Verification items for the finished model (mm, model axes). Face numbers are marked on the shaded views. Coordinates: 2 decimals unless noted, no trailing zeros. Loops run counter-clockwise (first coordinate to the right, second up) from the corner with the lowest first, then second, coordinate; pieces in that order, holes last. Notation, with made-up numbers: (8, 72) -> (18, 72) arc R12 ccw to (18, 84) -> close; hole circle Ø11 at (39, -9). An arc over 180 degrees is marked (long way). Use CSV: the item, a comma, the result in double quotes. Start each with the question number.
```python
from build123d import *

# Parameters (mm, degrees)
F2_R     = 12.7
F3_DEPTH = 31.801
F4_R     = 8
F5_DEPTH = 241.301


# Not quite as in the source:
# - a feature names something its author has since deleted; it is built from what else it names


with BuildPart() as f1:
    # F0 (on Front) → F1 (revolve)
    with BuildSketch(Plane.XZ):
        with BuildLine():
            ThreePointArc((164.1, 12.7), (167.8197438789, 3.7197438789), (176.8, 0))
            Line((176.8, 0), (241.3, 0))
            Line((241.3, 0), (241.3, 31.8))
            Line((241.3, 31.8), (187.2316558701, 31.8))
            ThreePointArc((187.2316558701, 31.8), (183.853704832, 33.1136133159), (182.2506823796, 36.3642212863))
            Line((182.2506823796, 36.3642212863), (180.9670874285, 51.0357787137))
            ThreePointArc((180.9670874285, 51.0357787137), (179.3640649761, 54.2863866841), (175.986113938, 55.6))
            Line((175.986113938, 55.6), (164.1, 55.6))
            Line((164.1, 55.6), (164.1, 12.7))
        make_face()
    revolve(axis=Axis((0, 0, 27.8), (0, 0, 1)))

    # F2 (on face) → F3 (cut, through all)
    with BuildSketch(Plane.XY.offset(31.8)):
        with Locations((-55.8790318376, 208.5433858958)):
            Circle(F2_R)
        with Locations((-152.6643540582, 152.6643540582)):
            Circle(F2_R)
        with Locations((-208.5433858958, 55.8790318376)):
            Circle(F2_R)
        with Locations((-208.5433858958, -55.8790318376)):
            Circle(F2_R)
        with Locations((-152.6643540582, -152.6643540582)):
            Circle(F2_R)
        with Locations((-55.8790318376, -208.5433858958)):
            Circle(F2_R)
        with Locations((55.8790318376, -208.5433858958)):
            Circle(F2_R)
        with Locations((152.6643540582, -152.6643540582)):
            Circle(F2_R)
        with Locations((208.5433858958, -55.8790318376)):
            Circle(F2_R)
        with Locations((208.5433858958, 55.8790318376)):
            Circle(F2_R)
        with Locations((152.6643540582, 152.6643540582)):
            Circle(F2_R)
        with Locations((55.8790318376, 208.5433858958)):
            Circle(F2_R)
    extrude(amount=-F3_DEPTH, mode=Mode.SUBTRACT)

    # F4 (on Front) → F5 (cut, through all)
    with BuildSketch(Plane.XZ):
        with Locations((0, 15.9)):
            Circle(F4_R)
    extrude(amount=F5_DEPTH, mode=Mode.SUBTRACT)


solid = f1.part
```
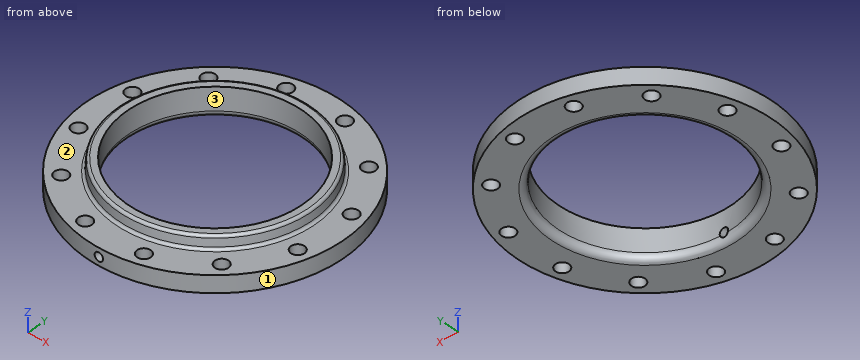
1. Release check for a two-part mould opening along X. For the marked faces 1, 2 and 3 record: released by +X, released by -X, zero draft, split by the parting line, or undercut.
2. Cross-section at B-B, the plane x = 0. Record the boundary of the cut face in (y, z), plus the area to 3 significant figures.
3. Cross-section at A-A, the plane y = 0. Record the boundary of the cut face in (x, z), plus the area to 3 significant figures.
4. Depth check by flat-ended pin: pin 1 (2 mm diameter, centred on y = 188.5, z = 30.5, fed in from -X); pin 2 (12 mm diameter, centred on x = -157.5, y = -99.5, fed in from +Z); pin 3 (3 mm diameter, centred on y = -150.5, z = 24, fed in from -X). Enter the tip coordinate at first touch or a pass-through.
5. Scan lines: line 1 (Y direction, x = -212, z = 8); line 2 (Z direction, x = 0, y = -214.5); line 3 (X direction, y = -49, z = 5.5). Record each from-to range of solid material in increasing order.
Solution:
1,face 1,"split by the parting line"
1,face 2,"zero draft"
1,face 3,"undercut"
2,outline,"(-241.3, 0) -> (-176.8, 0) arc R12.7 ccw to (-165.04, 7.9) -> (-241.3, 7.9) -> close; (-241.3, 23.9) -> (-164.1, 23.9) -> (-164.1, 55.6) -> (-175.99, 55.6) arc R5 ccw to (-180.97, 51.04) -> (-182.25, 36.36) arc R5 cw to (-187.23, 31.8) -> (-241.3, 31.8) -> close; (164.1, 12.7) arc R12.7 ccw to (176.8, 0) -> (241.3, 0) -> (241.3, 31.8) -> (187.23, 31.8) arc R5 cw to (182.25, 36.36) -> (180.97, 51.04) arc R5 ccw to (175.99, 55.6) -> (164.1, 55.6) -> close"
2,area,"4,440 mm2"
3,outline,"(-241.3, 0) -> (-176.8, 0) arc R12.7 ccw to (-164.1, 12.7) -> (-164.1, 55.6) -> (-175.99, 55.6) arc R5 ccw to (-180.97, 51.04) -> (-182.25, 36.36) arc R5 cw to (-187.23, 31.8) -> (-241.3, 31.8) -> close; (164.1, 12.7) arc R12.7 ccw to (176.8, 0) -> (241.3, 0) -> (241.3, 31.8) -> (187.23, 31.8) arc R5 cw to (182.25, 36.36) -> (180.97, 51.04) arc R5 ccw to (175.99, 55.6) -> (164.1, 55.6) -> close"
3,area,"5,670 mm2"
4,pin 1,"stops at x = -151.89"
4,pin 2,"stops at z = 53.13"
4,pin 3,"stops at x = -189.8"
5,line 1,"y = -115.25 to -68.1, -43.66 to 43.66, 68.1 to 115.25"
5,line 2,"z = 0 to 7.9, 23.9 to 31.8"
5,line 3,"x = -236.27 to -219.22, -197.87 to -158.96, 158.96 to 197.87, 219.22 to 236.27"
